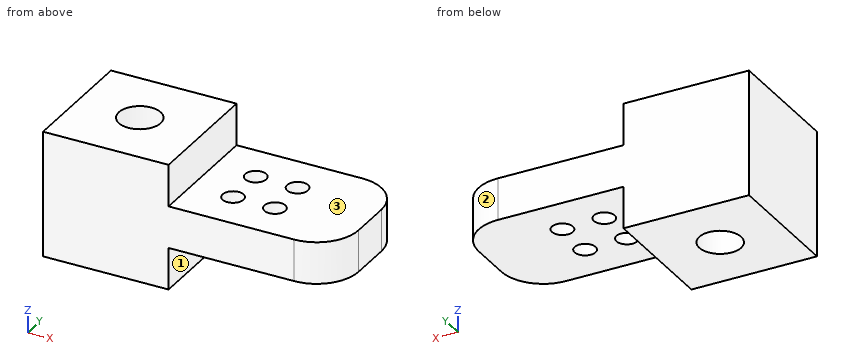
from build123d import *

# Parameters (mm, degrees)
F1_DEPTH = 38.1
F3_D     = 6.35
F5_D     = 12.7
F6_R     = 12.7


with BuildPart() as f1:
    # F0 (on Front) → F1 (new body)
    with BuildSketch(Plane.XZ):
        Polygon((0, 38.1), (0, 0), (38.1, 0), (38.1, 12.7), (88.9, 12.7), (88.9, 25.4), (38.1, 25.4), (38.1, 38.1), align=None)
    extrude(amount=-F1_DEPTH)

    # F3 (through all)
    with Locations(Plane.XY.offset(25.4)):
        with Locations((50.8, 25.4), (50.8, 12.7), (63.5, 12.7), (63.5, 25.4)):
            Hole(F3_D / 2)

    # F5 (through all)
    with Locations(Plane.XY.offset(38.1)):
        with Locations((19.05, 19.05)):
            Hole(F5_D / 2)

    # F6
    f6_edges = [f1.edges().sort_by_distance(p)[0] for p in [
        (88.9, 0, 19.05),
        (88.9, 38.1, 19.05),
    ]]
    fillet(f6_edges, radius=F6_R)


solid = f1.part
Build history of the part. All positions in model axes, mm. Face numbers are marked on the shaded views. A direction names the side the tool comes from. Coordinates: 2 decimals unless noted, no trailing zeros. Write each loop counter-clockwise with the first axis right and the second up, starting at its lowest first coordinate (ties: lowest second). Pieces come first, ordered by that corner, then holes.
(1) Cut at D-D on z = 21.5. List the corners of the cut face in (x, y) (3 decimals), and give its area (3 significant figures).
(2) Drill centre lines: line 1 (Y direction, x = 50.8, z = 17.5) (3 decimals); line 2 (Y direction, x = 19.05, z = 12.5); line 3 (Y direction, x = 63, z = 21). Where is each one in solid material? Low to high.
(3) Pin check, flat tips, straight feed: pin 1 Ø6.5 at (y, z) = (18.5, 31) entering from +X; pin 2 Ø10 at (x, z) = (59, 5) entering from -Y; pin 3 Ø6 at (x, y) = (67, 24) entering from +Z; pin 4 Ø10 at (x, y) = (55, 32) entering from -Z. Stop position of each tip, or through.
(4) Cut at A-A on x = 19.05. List the corners of the cut face in (y, z), and give its area (3 significant figures).
(5) Cut at C-C on x = 63.5. List the corners of the cut face in (y, z) (3 decimals), and give its area (3 significant figures).
(6) 3-axis set-ups, long thin cutter, end or side, ignore diameter. For the marked faces 1, 2 and 3: which of +Z, -Z, +X, -X, +Y, -Y reach the whole face in a straight line?
(7) Cut at B-B on y = 19.05. List the corners of the cut face in (x, z), and give its area (3 significant figures).
Working result:
1. outline: (0, 0) - (76.2, 0) arc R12.7 ccw to (88.9, 12.7) - (88.9, 25.4) arc R12.7 ccw to (76.2, 38.1) - (0, 38.1) - close; hole circle Ø12.7 at (19.05, 19.05); hole circle Ø6.35 at (50.8, 12.7); hole circle Ø6.35 at (50.8, 25.4); hole circle Ø6.35 at (63.5, 12.7); hole circle Ø6.35 at (63.5, 25.4)
1. area: 3,060 mm2
2. line 1: y = 0 to 9.525, 15.875 to 22.225, 28.575 to 38.1
2. line 2: y = 0 to 12.7, 25.4 to 38.1
2. line 3: y = 0 to 9.56, 15.84 to 22.26, 28.54 to 38.1
3. pin 1: stops at x = 38.1
3. pin 2: passes through
3. pin 3: stops at z = 25.4
3. pin 4: stops at z = 12.7
4. outline: (0, 0) - (12.7, 0) - (12.7, 38.1) - (0, 38.1) - close; (25.4, 0) - (38.1, 0) - (38.1, 38.1) - (25.4, 38.1) - close
4. area: 968 mm2
5. outline: (0, 12.7) - (9.525, 12.7) - (9.525, 25.4) - (0, 25.4) - close; (15.875, 12.7) - (22.225, 12.7) - (22.225, 25.4) - (15.875, 25.4) - close; (28.575, 12.7) - (38.1, 12.7) - (38.1, 25.4) - (28.575, 25.4) - close
5. area: 323 mm2
6. face 1: -Z, +X, +Y, -Y
6. face 2: +Z, -Z, +X, +Y
6. face 3: +Z, +X, +Y, -Y
7. outline: (0, 0) - (12.7, 0) - (12.7, 38.1) - (0, 38.1) - close; (25.4, 0) - (38.1, 0) - (38.1, 12.7) - (88.9, 12.7) - (88.9, 25.4) - (38.1, 25.4) - (38.1, 38.1) - (25.4, 38.1) - close
7. area: 1,610 mm2
